CAD build for the part. Positions are in the model's coordinates, mm. Give positions to 0.01 mm unless a question says otherwise; leave off trailing zeros. Loops run counter-clockwise (first coordinate to the right, second up) from the corner with the lowest first, then second, coordinate; pieces in that order, holes last.
```python
from build123d import *

# Parameters (mm, degrees)
IZIM1_R                     = 3.25
IZIM1_R_2                   = 0.725
Y_KSEKLIK_EKSTR_ZYON3_DEPTH = 0.5
IZIM2_R                     = 1.075
IZIM2_R_2                   = 0.375
IZIM2_R_3                   = 3.6
IZIM2_R_4                   = 2.9
KES_EKSTR_ZYON_NCE1_DEPTH   = 0.5


with BuildPart() as part:
    # Çizim1 → Yükseklik-Ekstrüzyon3 (new body)
    with BuildSketch(Plane.XY):
        with BuildLine():
            Line((-19.29792735, 2.8), (-16.75, 2.8))
            Line((-16.75, 2.8), (-16.75, 9.984362774))
            ThreePointArc((-16.75, 9.984362774), (-10.701322664, 16.301278884), (-2.5, 19.339079606))
            Line((-2.5, 19.339079606), (-2.5, 16.789079606))
            Line((-2.5, 16.789079606), (2.5, 16.789079606))
            Line((2.5, 16.789079606), (2.5, 19.339079606))
            ThreePointArc((2.5, 19.339079606), (10.701322664, 16.301278884), (16.75, 9.984362774))
            Line((16.75, 9.984362774), (16.75, 2.8))
            Line((16.75, 2.8), (19.29792735, 2.8))
            ThreePointArc((19.29792735, 2.8), (19.5, 0), (19.29792735, -2.8))
            Line((19.29792735, -2.8), (16.75, -2.8))
            Line((16.75, -2.8), (16.75, -9.984362774))
            ThreePointArc((16.75, -9.984362774), (10.701322664, -16.301278884), (2.5, -19.339079606))
            Line((2.5, -19.339079606), (2.5, -16.789079606))
            Line((2.5, -16.789079606), (-2.5, -16.789079606))
            Line((-2.5, -16.789079606), (-2.5, -19.339079606))
            ThreePointArc((-2.5, -19.339079606), (-10.701322664, -16.301278884), (-16.75, -9.984362774))
            Line((-16.75, -9.984362774), (-16.75, -2.8))
            Line((-16.75, -2.8), (-19.29792735, -2.8))
            ThreePointArc((-19.29792735, -2.8), (-19.5, 0), (-19.29792735, 2.8))
        make_face()
        with Locations((9.5, 0)):
            Circle(IZIM1_R, mode=Mode.SUBTRACT)
        with Locations((0, -9.939079606)):
            Circle(IZIM1_R_2, mode=Mode.SUBTRACT)
        with Locations(Location((-9.5, 0, 0), (0, 0, 180))):
            Circle(IZIM1_R, mode=Mode.SUBTRACT)
        with Locations((3, -9.939079606)):
            Circle(IZIM1_R_2, mode=Mode.SUBTRACT)
        with Locations((6, -9.939079606)):
            Circle(IZIM1_R_2, mode=Mode.SUBTRACT)
        with Locations((-3, -9.939079606)):
            Circle(IZIM1_R_2, mode=Mode.SUBTRACT)
        with Locations((-6, -9.939079606)):
            Circle(IZIM1_R_2, mode=Mode.SUBTRACT)
    extrude(amount=Y_KSEKLIK_EKSTR_ZYON3_DEPTH)

    # Çizim2 → Kes-Ekstrüzyon-İnce1 (cut)
    with BuildSketch(Plane.XY.offset(0.5)):
        with BuildLine():
            Line((-17.1, -10.080302575), (-17.1, -3.15))
            Line((-17.1, -3.15), (-19.598469328, -3.15))
            ThreePointArc((-19.598469328, -3.15), (-19.85, 0), (-19.598469328, 3.15))
            Line((-19.598469328, 3.15), (-17.1, 3.15))
            Line((-17.1, 3.15), (-17.1, 10.080302575))
            ThreePointArc((-17.1, 10.080302575), (-10.767327068, 16.675945785), (-2.15, 19.73322072))
            Line((-2.15, 19.73322072), (-2.15, 17.139079606))
            Line((-2.15, 17.139079606), (2.15, 17.139079606))
            Line((2.15, 17.139079606), (2.15, 19.73322072))
            ThreePointArc((2.15, 19.73322072), (10.767327068, 16.675945785), (17.1, 10.080302575))
            Line((17.1, 10.080302575), (17.1, 3.15))
            Line((17.1, 3.15), (19.598469328, 3.15))
            ThreePointArc((19.598469328, 3.15), (19.85, 0), (19.598469328, -3.15))
            Line((19.598469328, -3.15), (17.1, -3.15))
            Line((17.1, -3.15), (17.1, -10.080302575))
            ThreePointArc((17.1, -10.080302575), (10.767327068, -16.675945785), (2.15, -19.73322072))
            Line((2.15, -19.73322072), (2.15, -17.139079606))
            Line((2.15, -17.139079606), (-2.15, -17.139079606))
            Line((-2.15, -17.139079606), (-2.15, -19.73322072))
            ThreePointArc((-2.15, -19.73322072), (-10.767327068, -16.675945785), (-17.1, -10.080302575))
        make_face()
        with BuildLine():
            Line((-16.4, -9.887492099), (-16.4, -2.45))
            Line((-16.4, -2.45), (-18.99263015, -2.45))
            ThreePointArc((-18.99263015, -2.45), (-19.15, 0), (-18.99263015, 2.45))
            Line((-18.99263015, 2.45), (-16.4, 2.45))
            Line((-16.4, 2.45), (-16.4, 9.887492099))
            ThreePointArc((-16.4, 9.887492099), (-10.635451675, 15.925126928), (-2.85, 18.936736783))
            Line((-2.85, 18.936736783), (-2.85, 16.439079606))
            Line((-2.85, 16.439079606), (2.85, 16.439079606))
            Line((2.85, 16.439079606), (2.85, 18.936736783))
            ThreePointArc((2.85, 18.936736783), (10.635451675, 15.925126928), (16.4, 9.887492099))
            Line((16.4, 9.887492099), (16.4, 2.45))
            Line((16.4, 2.45), (18.99263015, 2.45))
            ThreePointArc((18.99263015, 2.45), (19.15, 0), (18.99263015, -2.45))
            Line((18.99263015, -2.45), (16.4, -2.45))
            Line((16.4, -2.45), (16.4, -9.887492099))
            ThreePointArc((16.4, -9.887492099), (10.635451675, -15.925126928), (2.85, -18.936736783))
            Line((2.85, -18.936736783), (2.85, -16.439079606))
            Line((2.85, -16.439079606), (-2.85, -16.439079606))
            Line((-2.85, -16.439079606), (-2.85, -18.936736783))
            ThreePointArc((-2.85, -18.936736783), (-10.635451675, -15.925126928), (-16.4, -9.887492099))
        make_face(mode=Mode.SUBTRACT)
        with Locations((-6, -9.939079606)):
            Circle(IZIM2_R)
        with Locations((-6, -9.939079606)):
            Circle(IZIM2_R_2, mode=Mode.SUBTRACT)
        with Locations((-3, -9.939079606)):
            Circle(IZIM2_R)
        with Locations((-3, -9.939079606)):
            Circle(IZIM2_R_2, mode=Mode.SUBTRACT)
        with Locations((6, -9.939079606)):
            Circle(IZIM2_R)
        with Locations((6, -9.939079606)):
            Circle(IZIM2_R_2, mode=Mode.SUBTRACT)
        with Locations((3, -9.939079606)):
            Circle(IZIM2_R)
        with Locations((3, -9.939079606)):
            Circle(IZIM2_R_2, mode=Mode.SUBTRACT)
        with Locations((-9.5, 0)):
            Circle(IZIM2_R_3)
        with Locations((-9.5, 0)):
            Circle(IZIM2_R_4, mode=Mode.SUBTRACT)
        with Locations((0, -9.939079606)):
            Circle(IZIM2_R)
        with Locations((0, -9.939079606)):
            Circle(IZIM2_R_2, mode=Mode.SUBTRACT)
        with Locations((9.5, 0)):
            Circle(IZIM2_R_3)
        with Locations((9.5, 0)):
            Circle(IZIM2_R_4, mode=Mode.SUBTRACT)
    extrude(amount=-KES_EKSTR_ZYON_NCE1_DEPTH, mode=Mode.SUBTRACT)


solid = part.part
```
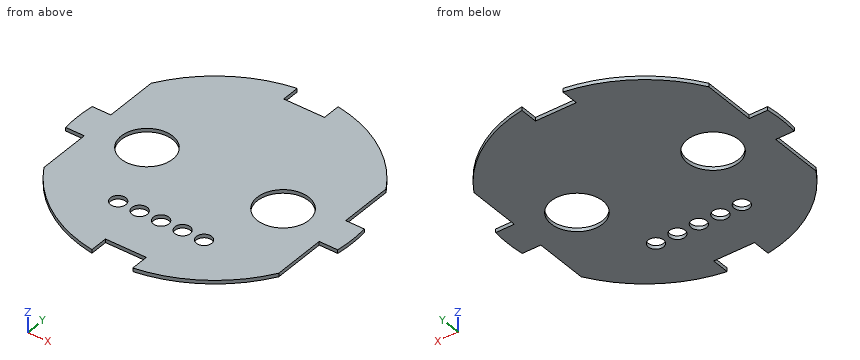
1. Saw through at B-B, the plane x = -12.5. List the corners of the cut face in (y, z).
Responses:
outline: (-14.51, 0) - (-1.99, 0) - (-1.99, 0.5) - (-14.51, 0.5) - close; (1.99, 0) - (14.51, 0) - (14.51, 0.5) - (1.99, 0.5) - close
2. Saw through at D-D, the plane y = -7. List the corners of the cut face in (x, z).
Responses:
outline: (-16.4, 0) - (16.4, 0) - (16.4, 0.5) - (-16.4, 0.5) - close
3. Saw through at C-C, the plane z = 0.35. Count the separate pieces of the cut face and the enclosed holes in it, and give its area (3 significant figures).
Responses:
separate pieces: 1
enclosed holes: 7
area: 975 mm2
4. Saw through at A-A, the plane y = 0. List the corners of the cut face in (x, z), and give its area (4 significant figures).
Responses:
outline: (-19.15, 0) - (-13.1, 0) - (-13.1, 0.5) - (-19.15, 0.5) - close; (-5.9, 0) - (5.9, 0) - (5.9, 0.5) - (-5.9, 0.5) - close; (13.1, 0) - (19.15, 0) - (19.15, 0.5) - (13.1, 0.5) - close
area: 11.95 mm2
5. Probe line 1 along X through (y, z) = (-10.5, 0.3); line 2 along Y through (x, z) = (9.5, 0.25); line 3 along Y through (x, z) = (16.5, 0.45). List the from-to ranges inside material, lowest first.
Responses:
line 1: x = -16.01 to -6.92, -5.08 to -3.92, -2.08 to -0.92, 0.92 to 2.08, 3.92 to 5.08, 6.92 to 16.01
line 2: y = -16.63 to -3.6, 3.6 to 16.63
line 3: y = -2.45 to 2.45
